from build123d import *

# Parameters (mm, degrees)
SKETCH2_R          = 1.3
CUT_EXTRUDE1_DEPTH = 7
SKETCH4_R          = 4.75
CUT_EXTRUDE2_DEPTH = 82.929848041
FILLET1_R          = 15
FILLET2_R          = 4


with BuildPart() as part:
    # Sketch1 → Revolve1 (revolve)
    with BuildSketch(Plane.XY, mode=Mode.PRIVATE) as revolve1_sk:
        Polygon((0, -40), (0, 40), (-12.5, 40), (-12.5, 37), (-8, 28), (-8, -28), (-12.5, -37), (-12.5, -40), align=None)
    revolve(revolve1_sk.sketch.rotate(Axis((0, -40, 0), (0, 1, 0)), 270), axis=Axis((0, -40, 0), (0, 1, 0)))

    # Sketch2 → Cut-Extrude1 (cut)
    with BuildSketch(Plane(origin=(0, 40, 0), x_dir=(1, 0, 0), z_dir=(0, 1, 0))):
        with Locations(Location((-6, 6, 0), (0, 0, 270))):
            Circle(SKETCH2_R)
        with Locations(Location((6, 6, 0), (0, 0, 270))):
            Circle(SKETCH2_R)
        with Locations(Location((-6, -6, 0), (0, 0, 270))):
            Circle(SKETCH2_R)
        with Locations(Location((6, -6, 0), (0, 0, 270))):
            Circle(SKETCH2_R)
    cut_extrude1 = extrude(amount=-CUT_EXTRUDE1_DEPTH, mode=Mode.SUBTRACT)

    # Mirror1: Cut-Extrude1 across plane
    add(cut_extrude1.mirror(Plane.ZX), mode=Mode.SUBTRACT)

    # Sketch3 → Cut-Revolve1 (revolve, cut)
    with BuildSketch(Plane(origin=(0, 0, 0), x_dir=(0, 0, -1), z_dir=(1, 0, 0))):
        Polygon((-7, 29.7), (0, 36.7), (0, -36.7), (-7, -29.7), align=None)
    revolve(axis=Axis((0, 36.7, 0), (0, -1, 0)), mode=Mode.SUBTRACT)

    # Sketch4 → Cut-Extrude2 (cut, through all)
    with BuildSketch(Plane(origin=(0, 40, 0), x_dir=(1, 0, 0), z_dir=(0, 1, 0))):
        with Locations(Location((0, 0, 0), (0, 0, 270))):
            Circle(SKETCH4_R)
    extrude(amount=-CUT_EXTRUDE2_DEPTH, mode=Mode.SUBTRACT)

    # Fillet1
    fillet1_edges = [part.edges().sort_by_distance(p)[0] for p in [
        (0, -28, 8),
        (0, 28, 8),
    ]]
    fillet(fillet1_edges, radius=FILLET1_R)

    # Fillet2
    fillet2_edges = [part.edges().sort_by_distance(p)[0] for p in [
        (0, 29.7, -7),
        (0, -29.7, -7),
    ]]
    fillet(fillet2_edges, radius=FILLET2_R)


solid = part.part
Could you check a few things on this model? Use its own coordinates, in mm. A direction names the side the tool comes from. Give positions to 0.01 mm unless a question says otherwise; leave off trailing zeros. Order: outer loops, then holes, each group sorted by start corner. A loop starts at its lowest first (then second) coordinate and runs counter-clockwise, first axis right, second up. Notation, with made-up numbers: (-14.5, 59) - (-5.5, 59) arc R25 ccw to (-5.5, 96) - close; hole circle Ø11 at (46.25, 84.5). An arc over 180 degrees is marked (long way). One line per item, written item: value. Start each with the question number.
1. For P1, Ø2, axis at x = -6, z = 6, coming from the -Y side; P2, Ø5, axis at y = -18.5, z = 2.5, coming from the +X side; P3, Ø5, axis at y = -30, z = -8, coming from the +X side, each with a flat end and sliding along its axis, tell me the tip position at first contact or that it passes through.
2. If I drill on probe 1 along X at (y, z) = (38, 6); probe 2 along X at (y, z) = (34.75, -6); probe 3 along Y at (x, z) = (7.25, 9.75), over which ranges is the centre line in solid material (lowest first)?
3. Imagine slicing it at A-A on y = -10.5. List the corners of the cut face in (x, z) for me, plus the area to 3 significant figures.
4. Thinking about a two-plate mould opening in Z: for faces 1 (the face through (6, 33, 6)), 2 (the face through (-2.921, 31.45, -9.276)), 3 (the face through (5, 40, 0)), which applies, +Z half, -Z half, draft (parallel to the pull), parting line (faces both ways), or undercut?
5. For faces 4 (the face through (-2.89, -35.92, -3.77)), 5 (the face through (-6, 33, 6)), 6 (the face through (-2.933, -31.532, -9.315)), 7 (the face through (-7.153, -36.549, 6.6)), which set-ups out of +Z, -Z, +X, -X, +Y, -Y let a thin tool reach every point of the face, with its end or its side?
Values:
1. P1: y = -33
1. P2: x = 8
1. P3: x = 7.69
2. probe 1: -10.97 to -7.3, -4.7 to 4.7, 7.3 to 10.97
2. probe 2: -9.66 to -7.3, -4.7 to 4.7, 7.3 to 9.66
2. probe 3: -40 to -36.3, 36.3 to 40
3. outline: circle Ø16 at (0, 0); hole circle Ø14 at (0, 0)
3. area: 47.1 mm²
4. face 1: undercut
4. face 2: parting line
4. face 3: draft
5. face 4: +Y, -Y
5. face 5: +Y
5. face 6: none
5. face 7: -Y
